Geometry: final body of the model. Coordinates: model frame, mm. A direction names the side the tool comes from. Round coordinates to 2 decimals unless told otherwise and drop trailing zeros. Order: outer loops, then holes, each group sorted by start corner. A loop starts at its lowest first (then second) coordinate and runs counter-clockwise, first axis right, second up. Notation, with made-up numbers: M 62,22 L 117,22 A14 cw 117,30 Z; hole C 53,84 d11. An arc over 180 degrees is marked long. Return JSON: item names as keys, results as strings. Group by question number.
Q1. Cut plane B-B on x = 0. Output: boundary loops of the cut face in (y, z).
Q2. Cut plane A-A on z = 38. Output: boundary loops of the cut face in (x, y), and give its area (3 significant figures).
Q3. Ray query, probe 1 along Y at (x, z) = (17, 40); probe 2 along Y at (x, z) = (2.5, -24.5); probe 3 along Z at (x, y) = (-27.5, 19.75). Return the intervals inside material, ascending.
Q4. Contact query for flat-ended pins moving along their axis: pin 1 (1.2 mm diameter, centred on y = 12.5, z = 44.5, fed in from +X); pin 2 (1.4 mm diameter, centred on x = -13, y = 13.5, fed in from +Z); pin 3 (12 mm diameter, centred on x = 0, z = -29.5, fed in from +Y). Output: stop coordinate, or through.
Q5. Cut plane C-C on y = 2.75. Output: boundary loops of the cut face in (x, z), and give its area (3 significant figures).
Q6. Mould query, pull axis X, two halves, no side actions, for faces 4 (the face through (4, 13, 43)), 5 (the face through (-31.439, 24.296, -0.609)), 6 (the face through (0.38, 1.711, 47.696)). Classes: released by +X, released by -X, zero draft, split by the parting line, or undercut.
Q7. Access query for faces 1 (the face through (0, 14.3, 43)), 2 (the face through (0, 25.6, -30)), 3 (the face through (-31.439, 13.149, -47.696)). Directions: +Z, -Z, +X, -X, +Y, -Y. A direction counts if a zero-diameter tool reaches every point of the face in a straight line with its end or side. Return the directions, or none.
Q8. Cut plane D-D on z = -17.5. Output: boundary loops of the cut face in (x, y).
```python
from build123d import *

# Parameters (mm, degrees)
SKETCH1_W           = 66.3
SKETCH1_H           = 26.1
BOSS_EXTRUDE1_DEPTH = 49.5
SKETCH2_R           = 3
SKETCH2_W           = 12.5
SKETCH2_H           = 4.6
SKETCH2_W_2         = 8
SKETCH2_H_2         = 2.5
CONNECTORS_DEPTH    = 13
SKETCH4_R           = 10
DISPLAY_DEPTH       = 0.5
FILLET1_R           = 6


with BuildPart() as part:
    # Sketch1 → Boss-Extrude1 (new, symmetric)
    with BuildSketch(Plane.XY):
        with Locations((0, 13.05)):
            Rectangle(SKETCH1_W, SKETCH1_H)
    extrude(amount=BOSS_EXTRUDE1_DEPTH, both=True)

    # Sketch2 → connectors (cut)
    with BuildSketch(Plane.XY.offset(49.5)):
        with Locations((17.15, 11.3)):
            Circle(SKETCH2_R)
        with Locations((-14.9, 13.05)):
            Rectangle(SKETCH2_W, SKETCH2_H)
        with Locations((0, 13.05)):
            Rectangle(SKETCH2_W_2, SKETCH2_H_2)
    extrude(amount=-CONNECTORS_DEPTH, mode=Mode.SUBTRACT)

    # Sketch4 → display (cut)
    with BuildSketch(Plane(origin=(0, 26.1, 0), x_dir=(1, 0, 0), z_dir=(0, 1, 0))):
        with Locations(Location((0, 29.5, 0), (0, 0, 270))):
            Circle(SKETCH4_R)
    extrude(amount=-DISPLAY_DEPTH, mode=Mode.SUBTRACT)

    # Fillet1
    fillet1_edges = [part.edges().sort_by_distance(p)[0] for p in [
        (33.15, 13.05, 49.5),
        (0, 26.1, 49.5),
        (-33.15, 13.05, 49.5),
        (0, 26.1, -49.5),
        (33.15, 13.05, -49.5),
        (0, 0, -49.5),
        (-33.15, 13.05, -49.5),
        (-33.15, 26.1, 0),
        (33.15, 26.1, 0),
        (33.15, 0, 0),
        (-33.15, 0, 0),
        (0, 0, 49.5),
    ]]
    fillet(fillet1_edges, radius=FILLET1_R)


solid = part.part
```
Result sheet:
{
 "1": {"outline": "M 0,-43.5 A6 ccw 6,-49.5 L 20.1,-49.5 A6 ccw 26.1,-43.5 L 26.1,-39.5 L 25.6,-39.5 L 25.6,-19.5 L 26.1,-19.5 L 26.1,43.5 A6 ccw 20.1,49.5 L 14.3,49.5 L 14.3,36.5 L 11.8,36.5 L 11.8,49.5 L 6,49.5 A6 ccw 0,43.5 Z"},
 "2": {"outline": "M -33.15,6 A6 ccw -27.15,0 L 27.15,0 A6 ccw 33.15,6 L 33.15,20.1 A6 ccw 27.15,26.1 L -27.15,26.1 A6 ccw -33.15,20.1 Z; hole M -21.15,10.75 L -8.65,10.75 L -8.65,15.35 L -21.15,15.35 Z; hole M -4,11.8 L 4,11.8 L 4,14.3 L -4,14.3 Z; hole C 17.15,11.3 d6", "area": "1,590 mm²"},
 "3": {"probe 1": "y = 0 to 8.3, 14.3 to 26.1", "probe 2": "y = 0 to 25.6", "probe 3": "z = -49.49 to 49.49"},
 "4": {"pin 1": "stops at x = 33.14", "pin 2": "stops at z = 36.5", "pin 3": "stops at y = 25.6"},
 "5": {"outline": "M -32.19,-43.5 A5.04 ccw -27.15,-48.54 L 27.15,-48.54 A5.04 ccw 32.19,-43.5 L 32.19,43.5 A5.04 ccw 27.15,48.54 L -27.15,48.54 A5.04 ccw -32.19,43.5 Z", "area": "6,230 mm²"},
 "6": {"face 4": "undercut", "face 5": "released by -X", "face 6": "zero draft"},
 "7": {"face 1": "+Z", "face 2": "+Y", "face 3": "-Z, -X, +Y, -Y"},
 "8": {"outline": "M -33.15,6 A6 ccw -27.15,0 L 27.15,0 A6 ccw 33.15,6 L 33.15,20.1 A6 ccw 27.15,26.1 L -27.15,26.1 A6 ccw -33.15,20.1 Z"}
}
